Part model, mm, in its own coordinate system. Give positions to 0.01 mm unless a question says otherwise; leave off trailing zeros. Order: outer loops, then holes, each group sorted by start corner. A loop starts at its lowest first (then second) coordinate and runs counter-clockwise, first axis right, second up. Notation, with made-up numbers: (-33.75, 60) - (-28.75, 60) arc R21 cw to (-28.75, 84) - close; hole circle Ø2 at (-17, 4.5). An arc over 180 degrees is marked (long way). Use a Markdown table: item, result. Add a question column.
from build123d import *

# Parameters (mm, degrees)
SKETCH_1_W             = 350
SKETCH_1_H             = 60
EXTRUDE_1_DEPTH        = 10
HOLE_WIZARD_M6_1_D     = 5
HOLE_WIZARD_M6_1_DEPTH = 20
HOLE_WIZARD_M6_1_TIP   = 1.502151548
MM_1_D                 = 12
MM_1_DEPTH             = 20
MM_1_TIP               = 3.605163714


with BuildPart() as part:
    # 草图1 → 凸台-拉伸1 (new body)
    with BuildSketch(Plane.XY):
        Rectangle(SKETCH_1_W, SKETCH_1_H)
    extrude(amount=EXTRUDE_1_DEPTH)

    # M6 螺纹孔1
    with Locations(Plane(origin=(-155, 0, 10), x_dir=(1, 0, 0), z_dir=(0, 0, 1))):
        with Locations((0, 0), (30, 0)):
            Hole(HOLE_WIZARD_M6_1_D / 2, depth=HOLE_WIZARD_M6_1_DEPTH)
            with Locations((0, 0, -(HOLE_WIZARD_M6_1_DEPTH + HOLE_WIZARD_M6_1_TIP / 2))):  # 118° drill point
                Cone(0, HOLE_WIZARD_M6_1_D / 2, HOLE_WIZARD_M6_1_TIP, mode=Mode.SUBTRACT)

    # 大小mm 暗销槽口1
    with Locations(Plane.XY.offset(10)):
        with Locations((155, -22.5), (155, 0), (155, 22.5)):
            Hole(MM_1_D / 2, depth=MM_1_DEPTH)
            with Locations((0, 0, -(MM_1_DEPTH + MM_1_TIP / 2))):  # 118° drill point
                Cone(0, MM_1_D / 2, MM_1_TIP, mode=Mode.SUBTRACT)


solid = part.part
1. Mould opens along X. For faces 1 (the face through (175, 0, 5)), 2 (the face through (159.76, -3.65, 4.93)), 3 (the face through (-2, 0, 10)), 4 (the face through (-175, 0, 5)) say: released by +X, released by -X, zero draft, split by the parting line, or undercut.
2. Cut at C-C (z = 4.25). Write the cut outline in (x, y).
3. Pin check, flat tip, straight feed: P1, Ø11, axis at x = 155, y = 22.5, coming from the +Z side. Stop position of the tip, or through.
4. Cut at A-A (y = -22.5). Write the cut outline in (x, z), plus the area to 3 significant figures.
5. Drill centre lines: probe 1 along Y at (x, z) = (155, 7); probe 2 along Y at (x, z) = (-155, 2); probe 3 along X at (y, z) = (-2, 3). Where is each one in solid material? Low to high. Write a range as [from, to].
6. Cut at B-B (x = 155). Write the cut outline in (y, z).
Responses:
| question | item | result |
|---|---|---|
| 1 | face 1 | released by +X |
| 1 | face 2 | undercut |
| 1 | face 3 | zero draft |
| 1 | face 4 | released by -X |
| 2 | outline | (-175, -30) - (175, -30) - (175, 30) - (-175, 30) - close; hole circle Ø5 at (-155, 0); hole circle Ø5 at (-125, 0); hole circle Ø12 at (155, -22.5); hole circle Ø12 at (155, 0); hole circle Ø12 at (155, 22.5) |
| 3 | P1 | passes through |
| 4 | outline | (-175, 0) - (149, 0) - (149, 10) - (-175, 10) - close; (161, 0) - (175, 0) - (175, 10) - (161, 10) - close |
| 4 | area | 3,380 mm² |
| 5 | probe 1 | y = [-30, -28.5], [-16.5, -6], [6, 16.5], [28.5, 30] |
| 5 | probe 2 | y = [-30, -2.5], [2.5, 30] |
| 5 | probe 3 | x = [-175, -156.5], [-153.5, -126.5], [-123.5, 149.34], [160.66, 175] |
| 6 | outline | (-30, 0) - (-28.5, 0) - (-28.5, 10) - (-30, 10) - close; (-16.5, 0) - (-6, 0) - (-6, 10) - (-16.5, 10) - close; (6, 0) - (16.5, 0) - (16.5, 10) - (6, 10) - close; (28.5, 0) - (30, 0) - (30, 10) - (28.5, 10) - close |
